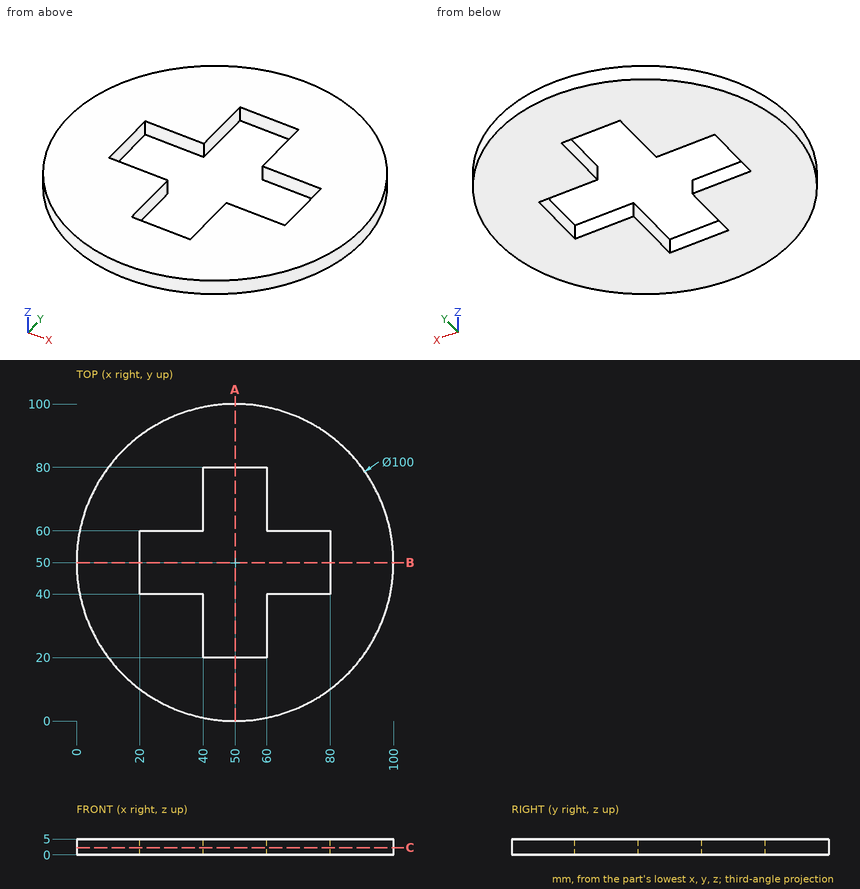
Design review of the part shown in the three views and the two pictorial views. Dimensions are in mm from the part's minimum x, y and z. Give positions to 0.01 mm unless a question says otherwise; leave off trailing zeros. Write each loop counter-clockwise with the first axis right and the second up, starting at its lowest first coordinate (ties: lowest second). Pieces come first, ordered by that corner, then holes. Notation, with made-up numbers: M -20,-28.5 L 19,-28.5 A22 cw 19,8.5 Z; hole C 7,41.5 d3. An arc over 180 degrees is marked long. Answer as CSV lines item,"result".
1. For pin 1 (1.5 mm diameter, centred on y = 63.5, z = 2.5, fed in from +X); pin 2 (1 mm diameter, centred on x = 61, z = 4.5, fed in from -Y); pin 3 (2.5 mm diameter, centred on x = 69, z = 2, fed in from +Y); pin 4 (2 mm diameter, centred on x = 89.5, y = 29.5, fed in from -Z), all flat-tipped, find the tip position at first contact; note any pin that passes through.
Findings:
pin 1,"stops at x = 98.35"
pin 2,"stops at y = 1.11"
pin 3,"stops at y = 96.74"
pin 4,"stops at z = 0"
2. Consider section A-A, the plane x = 50. Write out the cut boundary in (y, z), then the cut area to 3 significant figures.
Findings:
outline,"M 0,0 L 20,0 L 20,5 L 0,5 Z; M 80,0 L 100,0 L 100,5 L 80,5 Z"
area,"200 mm2"
3. Wall thickness on line 1 (Y direction, x = 50, z = 2.55); line 2 (X direction, y = 56, z = 3.2); line 3 (Y direction, x = 47, z = 3.6): over which ranges is each line inside the solid? List them lowest first.
Findings:
line 1,"y = 0 to 20, 80 to 100"
line 2,"x = 0.36 to 20, 80 to 99.64"
line 3,"y = 0.09 to 20, 80 to 99.91"
4. Consider section C-C, the plane z = 2.3. Write out the cut boundary in (x, y).
Findings:
outline,"C 50,50 d100; hole M 20,40 L 40,40 L 40,20 L 60,20 L 60,40 L 80,40 L 80,60 L 60,60 L 60,80 L 40,80 L 40,60 L 20,60 Z"
